```python
from build123d import *

# Parameters (mm, degrees)
EXTRUDE_1_DEPTH     = 6
BOSS_EXTRUDE4_DEPTH = 0.1


with BuildPart() as part:
    # Эскиз1 → Бобышка-Вытянуть1 (new body)
    with BuildSketch(Plane(origin=(0, 0, 0), x_dir=(0, 0, -1), z_dir=(1, 0, 0))):
        Polygon((0, 0), (100, 0), (60, 150), (0, 150), align=None)
    extrude(amount=EXTRUDE_1_DEPTH)

    # Sketch1 → Boss-Extrude4 (add)
    with BuildSketch(Plane.XZ):
        with BuildLine():
            Line((3, -27.25), (3, 0))
            Line((3, 0), (0, 0))
            Line((0, 0), (0, -48.591302246))
            Line((0, -48.591302246), (0.078671208, -48.591302246))
            Line((0.078671208, -48.591302246), (1.253102949, -28.895833333))
            ThreePointArc((1.253102949, -28.895833333), (1.799956598, -27.726266969), (3, -27.25))
        make_face()
        with BuildLine():
            Line((6, 0), (3, 0))
            Line((3, 0), (3, -27.25))
            ThreePointArc((3, -27.25), (4.200043402, -27.726266969), (4.746897051, -28.895833333))
            Line((4.746897051, -28.895833333), (5.921328792, -48.591302246))
            Line((5.921328792, -48.591302246), (6, -48.591302246))
            Line((6, -48.591302246), (6, 0))
        make_face()
        with BuildLine():
            Line((6, -100), (6, -50))
            ThreePointArc((6, -50), (5.121320344, -52.121320344), (3, -53))
            Line((3, -53), (3, -100))
            Line((3, -100), (6, -100))
        make_face()
        with BuildLine():
            ThreePointArc((3, -53), (0.878679656, -52.121320344), (0, -50))
            Line((0, -50), (0, -100))
            Line((0, -100), (3, -100))
            Line((3, -100), (3, -53))
        make_face()
    extrude(amount=BOSS_EXTRUDE4_DEPTH)


solid = part.part
```
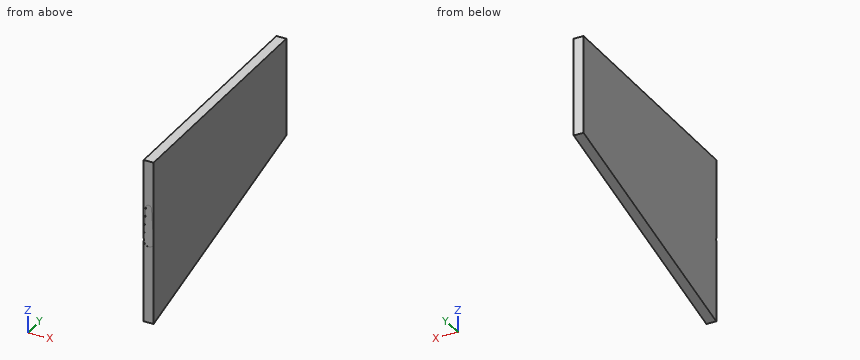
Input: part model. Units: mm. Frame: model coordinates. Coordinates: 2 decimals unless noted, no trailing zeros. Write each loop counter-clockwise with the first axis right and the second up, starting at its lowest first coordinate (ties: lowest second). Pieces come first, ordered by that corner, then holes. Notation, with made-up numbers: (34, 48) - (86, 48) arc R8 ccw to (86, 54) - close; hole circle Ø5 at (22.5, 80.5). An arc over 180 degrees is marked (long way). Put each result on its own line as item: value. Start each with the question number.
1) Cut plane B-B (y = 103.5). Return the cut outline in (x, z).
2) Ray query, L1, parallel to Y at x = 4.25, z = -47.5; L2, parallel to Z at x = 3.55, y = 77.5; L3, parallel to Z at x = 1.65, y = 24.5. Return the intervals inside material, ascending.
3) Contact query for flat-ended pins moving along their axis: pin 1 (3 mm diameter, centred on x = 3.5, z = -42, fed in from -Y); pin 2 (3 mm diameter, centred on x = 4, y = 73, fed in from -Z). Output: stop coordinate, or through.
4) Cut plane A-A (z = -72). Return the cut outline in (x, y), plus the area to 3 significant figures.
Resolved:
1. outline: (0, -72.4) - (6, -72.4) - (6, 0) - (0, 0) - close
2. L1: y = 0 to 150
2. L2: z = -79.33 to 0
2. L3: z = -93.47 to 0
3. pin 1: stops at y = 0
3. pin 2: stops at z = -80.93
4. outline: (0, -0.1) - (6, -0.1) - (6, 105) - (0, 105) - close
4. area: 631 mm2
